Work out the finished part from the listing and answer in its coordinate system (mm). A direction names the side the tool comes from. Round coordinates to 2 decimals unless told otherwise and drop trailing zeros. Write each loop counter-clockwise with the first axis right and the second up, starting at its lowest first coordinate (ties: lowest second). Pieces come first, ordered by that corner, then holes. Notation, with made-up numbers: (30, -12) -> (52, -12) arc R15 cw to (52, -8) -> close; hole circle Ø4 at (2, 38). An arc over 180 degrees is marked (long way). One line per item, written item: value.
```python
from build123d import *

# Parameters (mm, degrees)
SKETCH_1_W          = 5
SKETCH_1_H          = 30
EXTRUDE_1_DEPTH     = 7
EXTRUDE_1_2_DEPTH   = 7
SKETCH_2_R          = 2
CUT_EXTRUDE_1_DEPTH = 91.353769152
EXTRUDE_2_DEPTH     = 7


with BuildPart() as part:
    # Sketch 1 → Extrude 1 (new body)
    with BuildSketch(Plane(origin=(0, 0, 0), x_dir=(1, 0, 0), z_dir=(0, 1, 0))):
        with Locations((-39.97, 15)):
            Rectangle(SKETCH_1_W, SKETCH_1_H)
    extrude(amount=EXTRUDE_1_DEPTH)


with BuildPart() as body_2:
    # Sketch 1 → Extrude 1 2 (new body)
    with BuildSketch(Plane(origin=(0, 0, 0), x_dir=(1, 0, 0), z_dir=(0, 1, 0))):
        with Locations((39.97, 15)):
            Rectangle(SKETCH_1_W, SKETCH_1_H)
    extrude(amount=EXTRUDE_1_2_DEPTH)


with BuildPart() as cut_extrude_1_tool:
    # Sketch 2 → Cut-Extrude 1 (new, through all)
    with BuildSketch(Plane.ZY.offset(42.47)):
        with Locations((-15, 3.5)):
            Circle(SKETCH_2_R)
        with Locations((-25.033065305, 3.407092775)):
            Circle(SKETCH_2_R)
    extrude(amount=-CUT_EXTRUDE_1_DEPTH)


with BuildPart() as part_1:
    add(part.part)

    # Cut-Extrude 1: cut by cut_extrude_1_tool
    add(cut_extrude_1_tool.part, mode=Mode.SUBTRACT)



with BuildPart() as body_2_1:
    add(body_2.part)

    # Cut-Extrude 1: cut by cut_extrude_1_tool
    add(cut_extrude_1_tool.part, mode=Mode.SUBTRACT)


with BuildPart() as part_2:
    add(part_1.part)

    add(body_2_1.part)  # Extrude 2 merges body 2
    # Sketch 3 → Extrude 2 (add)
    with BuildSketch(Plane(origin=(0, 7, 0), x_dir=(1, 0, 0), z_dir=(0, 1, 0))):
        with BuildLine():
            ThreePointArc((22.449964365, -30), (25.304076717, -27.635205835), (27.910587597, -25))
            Line((27.910587597, -25), (-27.910587597, -25))
            ThreePointArc((-27.910587597, -25), (-25.304076717, -27.635205835), (-22.449964365, -30))
            Line((-22.449964365, -30), (22.449964365, -30))
        make_face()
        with BuildLine():
            ThreePointArc((-22.449964365, -30), (-25.304076717, -27.635205835), (-27.910587597, -25))
            ThreePointArc((-27.910587597, -25), (-34.99864724, -13.382660101), (-37.47, 0))
            Line((-37.47, 0), (-42.47, 0))
            ThreePointArc((-42.47, 0), (-39.245495492, -16.232436156), (-30.061618386, -30))
            Line((-30.061618386, -30), (-22.449964365, -30))
        make_face()
        with BuildLine():
            ThreePointArc((37.47, 0), (34.99864724, -13.382660101), (27.910587597, -25))
            ThreePointArc((27.910587597, -25), (25.304076717, -27.635205835), (22.449964365, -30))
            Line((22.449964365, -30), (30.061618386, -30))
            ThreePointArc((30.061618386, -30), (39.245495492, -16.232436156), (42.47, 0))
            Line((42.47, 0), (37.47, 0))
        make_face()
    extrude(amount=-EXTRUDE_2_DEPTH)


solid = part_2.part
```
(1) For a pull along Z with two mould halves and no side action, classify faces 3 (the face through (0, 0, 27)), 4 (the face through (35.07, 3.55, 13.2)), 5 (the face through (39.9, 2.3, -16.6)) as pulls with the +Z half, pulls with the -Z half, needs draft (parallel to the pull), parting line crosses it, or undercut.
Reported:
face 3: needs draft
face 4: pulls with the -Z half
face 5: undercut
(2) A flat-ended cylindrical pin translates along its axis: pin 1 Ø2 at (x, y) = (-6.5, 4) entering from -Z. Find the tip coordinate at first contact, or state that the pin passes through.
Reported:
pin 1: stops at z = 25
(3) Find section B-B on y = 4.5. Give the vertices of the cut face in (x, z), plus the area to 3 significant figures.
Reported:
outline: (-42.47, -30) -> (-37.47, -30) -> (-37.47, -26.71) -> (-42.47, -26.71) -> close; (-42.47, -23.36) -> (-37.47, -23.36) -> (-37.47, -16.73) -> (-42.47, -16.73) -> close; (-42.47, -13.27) -> (-37.47, -13.27) -> (-37.47, 0) arc R37.47 cw to (-27.91, 25) -> (27.91, 25) arc R37.47 cw to (37.47, 0) -> (37.47, -13.27) -> (42.47, -13.27) -> (42.47, 0) arc R42.47 ccw to (30.06, 30) -> (-30.06, 30) arc R42.47 ccw to (-42.47, 0) -> close; (37.47, -30) -> (42.47, -30) -> (42.47, -26.71) -> (37.47, -26.71) -> close; (37.47, -23.36) -> (42.47, -23.36) -> (42.47, -16.73) -> (37.47, -16.73) -> close
area: 825 mm2
(4) Consider probe 1 along Y at (x, z) = (-39.45, -15); probe 2 along X at (y, z) = (4.5, -13); probe 3 along Z at (x, y) = (-7, 2). Determine where each line is inside the solid, lowest interval first.
Reported:
probe 1: y = 0 to 1.5, 5.5 to 7
probe 2: x = -42.47 to -37.47, 37.47 to 42.47
probe 3: z = 25 to 30
(5) Find section A-A on z = -15. Give the vertices of the cut face in (x, y), plus the area to 3 significant figures.
Reported:
outline: (-42.47, 0) -> (-37.47, 0) -> (-37.47, 1.5) -> (-42.47, 1.5) -> close; (-42.47, 5.5) -> (-37.47, 5.5) -> (-37.47, 7) -> (-42.47, 7) -> close; (37.47, 0) -> (42.47, 0) -> (42.47, 1.5) -> (37.47, 1.5) -> close; (37.47, 5.5) -> (42.47, 5.5) -> (42.47, 7) -> (37.47, 7) -> close
area: 30.0 mm2
(6) Find section C-C on z = 19. Give the vertices of the cut face in (x, y).
Reported:
outline: (-37.98, 0) -> (-32.3, 0) -> (-32.3, 7) -> (-37.98, 7) -> close; (32.3, 0) -> (37.98, 0) -> (37.98, 7) -> (32.3, 7) -> close
(7) A tool of negligible diameter and unlimited length cuts with its end or side. For faces 1 (the face through (0, 4, 30)), 2 (the face through (-34.93, 3.55, 13.56)), from which of +Z, -Z, +X, -X, +Y, -Y can it reach the whole face along a straight path? Write none if from no direction.
Reported:
face 1: +Z, +X, -X, +Y, -Y
face 2: -Z, +Y, -Y
(8) Find section D-D on x = -25.5. Give the vertices of the cut face in (y, z).
Reported:
outline: (0, 25) -> (7, 25) -> (7, 30) -> (0, 30) -> close
